Work out the finished part from the listing and answer in its coordinate system (mm). Face numbers are marked on the shaded views. A direction names the side the tool comes from. Round coordinates to 2 decimals unless told otherwise and drop trailing zeros. Loops run counter-clockwise (first coordinate to the right, second up) from the corner with the lowest first, then second, coordinate; pieces in that order, holes last. Notation, with made-up numbers: (-22.5, 45.5) -> (12.5, 45.5) arc R11 cw to (12.5, 54.5) -> close; hole circle Ø3 at (-6.75, -35.5). An arc over 180 degrees is marked (long way). Use CSV: the item, a comma, the result in double quotes. Start each with the question number.
from build123d import *

# Parameters (mm, degrees)
SKETCH_1_W           = 145
SKETCH_1_H           = 90
EXTRUDE_1_DEPTH      = 10
SKETCH_2_W           = 125.8
SKETCH_2_H           = 90
EXTRUDE_2_DEPTH      = 3
SKETCH_3_W           = 123.8
SKETCH_3_H           = 88
CUT_EXTRUDE_1_DEPTH  = 3
CUT_EXTRUDE_2_DEPTH  = 3.5
SKETCH_6_W           = 141
SKETCH_6_H           = 86
CUT_EXTRUDE_3_DEPTH  = 4
SKETCH_7_W           = 36
SKETCH_7_H           = 6
CUT_EXTRUDE_4_DEPTH  = 153.377819908
SKETCH_8_W           = 7
SKETCH_8_H           = 86
CUT_EXTRUDE_5_DEPTH  = 4
EXTRUDE_6_DEPTH      = 4
EXTRUDE_7_DEPTH      = 4
EXTRUDE_8_DEPTH      = 0.1
EXTRUDE_8_DEPTH_BACK = 6.1
SKETCH_16_R          = 2.75
SKETCH_17_R          = 1.5
CUT_EXTRUDE_8_DEPTH  = 86.925898308
SKETCH_18_R          = 2.4
CUT_EXTRUDE_9_DEPTH  = 86.914201387
SKETCH_19_W          = 17
SKETCH_19_H          = 2.7
CUT_EXTRUDE_10_DEPTH = 3


with BuildPart() as part:
    # Эскиз1 → Бобышка-Вытянуть1 (new body)
    with BuildSketch(Plane(origin=(0, 0, 0), x_dir=(1, 0, 0), z_dir=(0, 1, 0))):
        Rectangle(SKETCH_1_W, SKETCH_1_H)
    extrude(amount=EXTRUDE_1_DEPTH)

    # Эскиз2 → Бобышка-Вытянуть2 (add)
    with BuildSketch(Plane(origin=(0, 10, 0), x_dir=(1, 0, 0), z_dir=(0, 1, 0))):
        Rectangle(SKETCH_2_W, SKETCH_2_H)
    extrude(amount=EXTRUDE_2_DEPTH)

    # Эскиз3 → Вырез-Вытянуть1 (cut)
    with BuildSketch(Plane(origin=(0, 13, 0), x_dir=(1, 0, 0), z_dir=(0, 1, 0))):
        Rectangle(SKETCH_3_W, SKETCH_3_H)
    extrude(amount=-CUT_EXTRUDE_1_DEPTH, mode=Mode.SUBTRACT)

    # Эскиз4 → Вырез-Вытянуть2 (cut)
    with BuildSketch(Plane(origin=(0, 10, 0), x_dir=(1, 0, 0), z_dir=(0, 1, 0))):
        with BuildLine():
            Line((-53.9, 43), (53.9, 43))
            Line((53.9, 43), (53.9, 40))
            ThreePointArc((53.9, 40), (55.071572875, 37.171572875), (57.9, 36))
            Line((57.9, 36), (60.9, 36))
            Line((60.9, 36), (60.9, -36))
            Line((60.9, -36), (57.9, -36))
            ThreePointArc((57.9, -36), (55.071572875, -37.171572875), (53.9, -40))
            Line((53.9, -40), (53.9, -43))
            Line((53.9, -43), (-53.9, -43))
            Line((-53.9, -43), (-53.9, -40))
            ThreePointArc((-53.9, -40), (-55.071572875, -37.171572875), (-57.9, -36))
            Line((-57.9, -36), (-60.9, -36))
            Line((-60.9, -36), (-60.9, 36))
            Line((-60.9, 36), (-57.9, 36))
            ThreePointArc((-57.9, 36), (-55.071572875, 37.171572875), (-53.9, 40))
            Line((-53.9, 40), (-53.9, 43))
        make_face()
    extrude(amount=-CUT_EXTRUDE_2_DEPTH, mode=Mode.SUBTRACT)

    # Эскиз6 → Вырез-Вытянуть3 (cut)
    with BuildSketch(Plane.XZ):
        Rectangle(SKETCH_6_W, SKETCH_6_H)
    extrude(amount=-CUT_EXTRUDE_3_DEPTH, mode=Mode.SUBTRACT)

    # Эскиз7 → Вырез-Вытянуть4 (cut, through all)
    with BuildSketch(Plane(origin=(72.5, 0, 0), x_dir=(0, 0, -1), z_dir=(1, 0, 0))):
        with Locations((0, 1)):
            Rectangle(SKETCH_7_W, SKETCH_7_H)
    extrude(amount=-CUT_EXTRUDE_4_DEPTH, mode=Mode.SUBTRACT)

    # Эскиз8 → Вырез-Вытянуть5 (cut)
    with BuildSketch(Plane.XZ.offset(-4)):
        with Locations((-67, 0)):
            Rectangle(SKETCH_8_W, SKETCH_8_H)
        with Locations((67, 0)):
            Rectangle(SKETCH_8_W, SKETCH_8_H)
    extrude(amount=-CUT_EXTRUDE_5_DEPTH, mode=Mode.SUBTRACT)

    # Эскиз14 → Бобышка-Вытянуть6 (add)
    with BuildSketch(Plane.XZ.offset(-4)):
        Polygon((-63.5, -37), (-63.5, -18), (63.5, -18), (63.5, -37), (61.5, -37), (61.5, -20), (14.5, -20), (14.5, -43), (12.5, -43), (12.5, -20), (-12.5, -20), (-12.5, -43), (-14.5, -43), (-14.5, -20), (-61.5, -20), (-61.5, -37), align=None)
    extrude(amount=EXTRUDE_6_DEPTH)

    # Эскиз15 → Бобышка-Вытянуть7 (add)
    with BuildSketch(Plane.XZ.offset(-4)):
        Polygon((-61.5, 37), (-63.5, 37), (-63.5, 18), (-50.5, 18), (-50.5, 43), (-55.5, 43), (-55.5, 20), (-61.5, 20), align=None)
        Polygon((63.5, 37), (63.5, 18), (50.5, 18), (50.5, 43), (55.5, 43), (55.5, 20), (61.5, 20), (61.5, 37), align=None)
        Polygon((-13.5, 43), (-13.5, 18), (13.5, 18), (13.5, 43), (8.5, 43), (8.5, 20), (-8.5, 20), (-8.5, 43), align=None)
    extrude(amount=EXTRUDE_7_DEPTH)

    # Эскиз16 → Бобышка-Вытянуть8 (add, two sides: drawn at the far end of the back side and taken through both)
    with BuildSketch(Plane(origin=(0, 10, 0), x_dir=(1, 0, 0), z_dir=(0, 1, 0)).offset(-EXTRUDE_8_DEPTH_BACK)):
        with Locations(Location((-57.5, 40, 0), (0, 0, 270))):
            Circle(SKETCH_16_R)
        with Locations(Location((57.5, 40, 0), (0, 0, 270))):
            Circle(SKETCH_16_R)
        with Locations(Location((-57.5, -40, 0), (0, 0, 270))):
            Circle(SKETCH_16_R)
        with Locations(Location((57.5, -40, 0), (0, 0, 270))):
            Circle(SKETCH_16_R)
    extrude(amount=EXTRUDE_8_DEPTH + EXTRUDE_8_DEPTH_BACK)

    # Эскиз17 → Вырез-Вытянуть8 (cut, through all)
    with BuildSketch(Plane(origin=(0, 10.1, 0), x_dir=(1, 0, 0), z_dir=(0, 1, 0))):
        with Locations(Location((-57.5, 40, 0), (0, 0, 270))):
            Circle(SKETCH_17_R)
        with Locations(Location((57.5, 40, 0), (0, 0, 270))):
            Circle(SKETCH_17_R)
        with Locations(Location((-57.5, -40, 0), (0, 0, 270))):
            Circle(SKETCH_17_R)
        with Locations(Location((57.5, -40, 0), (0, 0, 270))):
            Circle(SKETCH_17_R)
    extrude(amount=-CUT_EXTRUDE_8_DEPTH, mode=Mode.SUBTRACT)

    # Эскиз18 → Вырез-Вытянуть9 (cut, through all)
    with BuildSketch(Plane(origin=(0, 10, 0), x_dir=(1, 0, 0), z_dir=(0, 1, 0))):
        with Locations(Location((-67.5, 35, 0), (0, 0, 270))):
            Circle(SKETCH_18_R)
        with Locations(Location((-67.5, -35, 0), (0, 0, 270))):
            Circle(SKETCH_18_R)
        with Locations(Location((67.5, 35, 0), (0, 0, 270))):
            Circle(SKETCH_18_R)
        with Locations(Location((67.5, -35, 0), (0, 0, 270))):
            Circle(SKETCH_18_R)
    extrude(amount=-CUT_EXTRUDE_9_DEPTH, mode=Mode.SUBTRACT)

    # Эскиз19 → Вырез-Вытянуть10 (cut)
    with BuildSketch(Plane(origin=(0, 0, -45), x_dir=(-1, 0, 0), z_dir=(0, 0, -1))):
        with Locations((43.4, 12.65)):
            Rectangle(SKETCH_19_W, SKETCH_19_H)
    extrude(amount=-CUT_EXTRUDE_10_DEPTH, mode=Mode.SUBTRACT)


solid = part.part
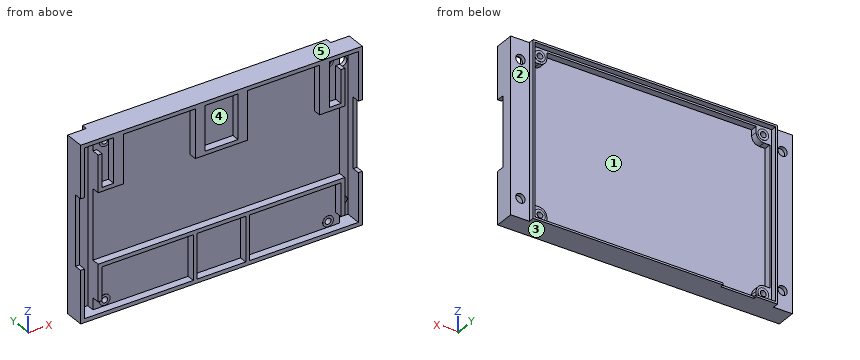
Q1. Section D-D, the plane x = -31 is taken. Write down the section's boundary in (y, z).
Q2. Each of these flat-tipped pins is pushed along its axis until it touches: pin 1 (3 mm diameter, centred on x = 40, z = 34.5, fed in from -Y); pin 2 (4.5 mm diameter, centred on x = 57, z = -39, fed in from +Y); pin 3 (3 mm diameter, centred on x = -15.5, z = -4, fed in from +Y). Where does it stop, or does it pass through?
Q3. Section B-B, the plane y = 2 is taken. Give the number of separate pieces and of enclosed holes in the cut face, and give its area (3 significant figures).
Q4. Section C-C, the plane z = -8 is taken. Write down the section's boundary in (x, y).
Q5. Section A-A, the plane x = 67.5 is taken. Write down the section's boundary in (y, z), and give its area (3 significant figures).
Q6. Straight lines are drawn through the part: line 1 (X direction, y = 5.75, z = -40); line 2 (X direction, y = 7, z = -40); line 3 (Z direction, x = -18, y = 2). For each, find the intervals that lie inside material, in ascending order. Write a range as from..to.
Q7. Which of the six approach directions +Z, -Z, +X, -X, +Y, -Y give full straight-line access (tool end or side, diameter ignored) to the marked faces 4 and 5?
Q8. For a pull along Z with two mould halves and no side action, classify the marked faces 1, 2 and 3 as pulls with the +Z half, pulls with the -Z half, needs draft (parallel to the pull), parting line crosses it, or undercut.
Report:
1,outline,"(0, -45) -> (13, -45) -> (13, -44) -> (10, -44) -> (10, -43) -> (6.5, -43) -> (6.5, 43) -> (10, 43) -> (10, 44) -> (13, 44) -> (13, 45) -> (0, 45) -> (0, 43) -> (4, 43) -> (4, -18) -> (0, -18) -> (0, -20) -> (4, -20) -> (4, -43) -> (0, -43) -> close"
2,pin 1,"stops at y = 4"
2,pin 2,"stops at y = 10.1"
2,pin 3,"stops at y = 6.5"
3,separate pieces,"2"
3,enclosed holes,"2"
3,area,"1,830 mm²"
4,outline,"(-72.5, 4) -> (-70.5, 4) -> (-70.5, 8) -> (-63.5, 8) -> (-63.5, 4) -> (63.5, 4) -> (63.5, 8) -> (70.5, 8) -> (70.5, 4) -> (72.5, 4) -> (72.5, 10) -> (62.9, 10) -> (62.9, 13) -> (61.9, 13) -> (61.9, 10) -> (60.9, 10) -> (60.9, 6.5) -> (-60.9, 6.5) -> (-60.9, 10) -> (-61.9, 10) -> (-61.9, 13) -> (-62.9, 13) -> (-62.9, 10) -> (-72.5, 10) -> close"
5,outline,"(0, -45) -> (10, -45) -> (10, -37.4) -> (8, -37.4) -> (8, -43) -> (0, -43) -> close; (0, 43) -> (8, 43) -> (8, 37.4) -> (10, 37.4) -> (10, 45) -> (0, 45) -> close; (8, -32.6) -> (10, -32.6) -> (10, 32.6) -> (8, 32.6) -> close"
5,area,"193 mm²"
6,line 1,"x = -72.5..-70.5, -63.5..-59, -56..56, 59..63.5, 70.5..72.5"
6,line 2,"x = -72.5..-70.5, -63.5..-59, -56..-53.9, 53.9..56, 59..63.5, 70.5..72.5"
6,line 3,"z = -45..-43, -20..-18, 43..45"
7,face 4,"-Y"
7,face 5,"+Z, +X, -X, +Y, -Y"
8,face 1,"undercut"
8,face 2,"needs draft"
8,face 3,"pulls with the -Z half"
